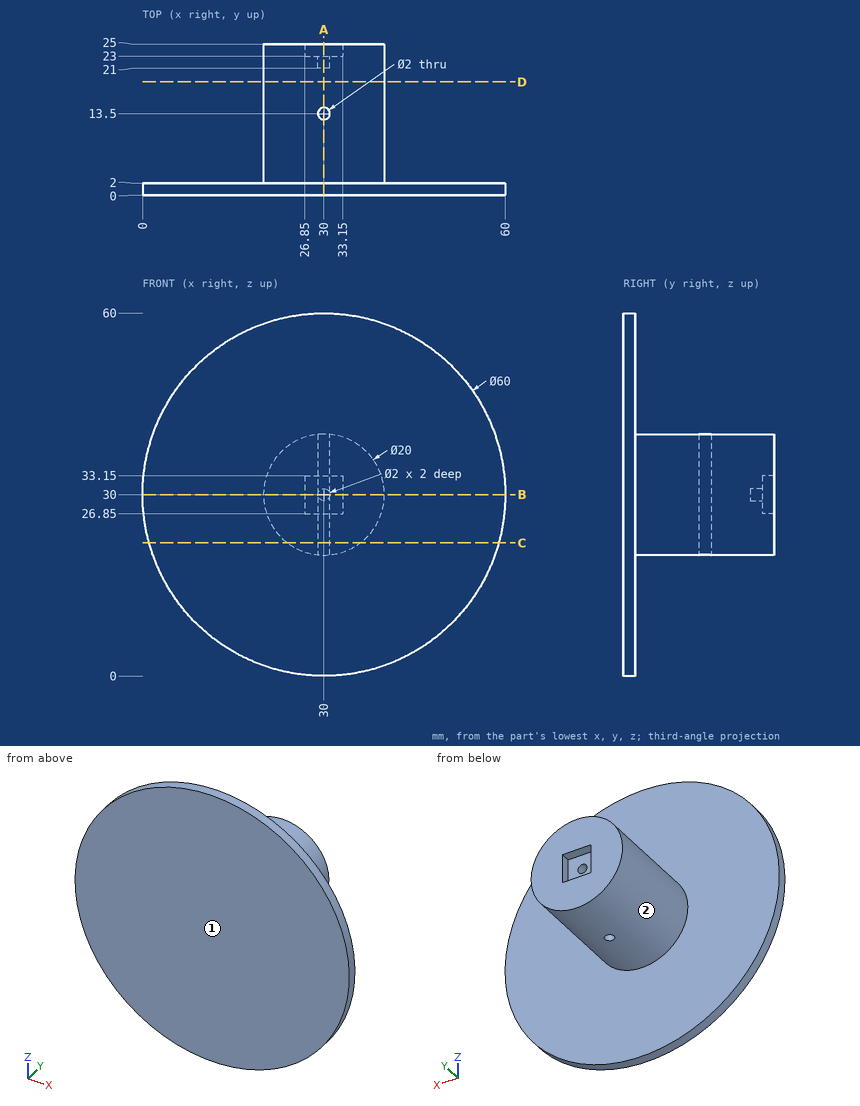
Geometry: see drawing. Coordinates: mm, zero at the bounding-box minimum. A direction names the side the tool comes from. Coordinates: 2 decimals unless noted, no trailing zeros. Write each loop counter-clockwise with the first axis right and the second up, starting at its lowest first coordinate (ties: lowest second). Pieces come first, ordered by that corner, then holes. Notation, with made-up numbers: (-9, 25) - (25, 25) arc R21 cw to (25, 52) - close; hole circle Ø9 at (58.25, 32). An arc over 180 degrees is marked (long way). Put each result on its own line as item: value. Start each with the question number.
1) Reachability of the marked faces 1 and 2 from +Z, -Z, +X, -X, +Y, -Y: full face, straight path, thin tool, end or side. Return the list, or none.
2) Cut plane D-D (y = 18.75). Return the cut outline in (x, z).
3) Cut plane B-B (z = 30). Return the cut outline in (x, y).
4) Ray query, L1, parallel to Y at x = 30, z = 28.5; L2, parallel to X at y = 21.7, z = 30; L3, parallel to Y at x = 30, z = 26. Return the intervals inside material, ascending.
5) Cut plane A-A (x = 30). Return the cut outline in (y, z).
6) Cut plane C-C (z = 22). Return the cut outline in (x, y).
7) Contact query for flat-ended pins moving along their axis: pin 1 (1.6 mm diameter, centred on x = 29.5, y = 24.5, fed in from +Z); pin 2 (6 mm diameter, centred on y = 11, z = 42, fed in from -X); pin 3 (2 mm diameter, centred on y = 24.5, z = 31.5, fed in from +X). Output: stop coordinate, or through.
Resolved:
1. face 1: +Z, -Z, +X, -X, -Y
1. face 2: +Y
2. outline: circle Ø20 at (30, 30)
3. outline: (0, 0) - (60, 0) - (60, 2) - (40, 2) - (40, 25) - (33.15, 25) - (33.15, 23) - (31, 23) - (31, 21) - (29, 21) - (29, 23) - (26.85, 23) - (26.85, 25) - (20, 25) - (20, 2) - (0, 2) - close; hole circle Ø2 at (30, 13.5)
4. L1: y = 0 to 12.5, 14.5 to 23
4. L2: x = 20 to 29, 31 to 40
4. L3: y = 0 to 12.5, 14.5 to 25
5. outline: (0, 0) - (2, 0) - (2, 20) - (12.5, 20) - (12.5, 40) - (2, 40) - (2, 60) - (0, 60) - close; (14.5, 20) - (25, 20) - (25, 26.85) - (23, 26.85) - (23, 29) - (21, 29) - (21, 31) - (23, 31) - (23, 33.15) - (25, 33.15) - (25, 40) - (14.5, 40) - close
6. outline: (1.09, 0) - (58.91, 0) - (58.91, 2) - (36, 2) - (36, 25) - (24, 25) - (24, 2) - (1.09, 2) - close; hole circle Ø2 at (30, 13.5)
7. pin 1: stops at z = 40
7. pin 2: stops at x = 25.64
7. pin 3: stops at x = 39.99
